Build history of the part. All positions in model axes, mm. A direction names the side the tool comes from. Give positions to 0.01 mm unless a question says otherwise; leave off trailing zeros. Loops run counter-clockwise (first coordinate to the right, second up) from the corner with the lowest first, then second, coordinate; pieces in that order, holes last. Notation, with made-up numbers: (-38.5, 55) - (-26.5, 55) arc R18 ccw to (-26.5, 60) - close; hole circle Ø1 at (-27, 7). An arc over 180 degrees is marked (long way). Return JSON: item names as keys, results as strings. Group by question number.
1) 3-axis set-ups, long thin cutter, end or side, ignore diameter. For faces 4 (the face through (-1, 2.641, 64)), 5 (the face through (39.531, 0, 40)), 6 (the face through (-1, -6.109, 40)), 7 (the face through (-1, 6.109, 40)), 8 (the face through (-39.531, 0, 40)): which of +Z, -Z, +X, -X, +Y, -Y reach the whole face in a straight line?
2) Slice it at D-D (x = 0). List the corners of the cut face in (y, z).
3) Drop flat-ended pins along their axis: pin 1 (3 mm diameter, centred on x = -2.5, z = 21.5, fed in from +Y); pin 2 (13.5 mm diameter, centred on y = -1, z = 37, fed in from +X); pin 3 (1.5 mm diameter, centred on y = -23.5, z = 7, fed in from -X); pin 4 (7 mm diameter, centred on x = -21.57, z = 27.49, fed in from -Y). Give the stop position or say it passes through.
4) Slice it at A-A (x = -17.5). List the corners of the cut face in (y, z).
5) Mould opens along Z. For faces 1 (the face through (-17.1, 0.1, 31.5)), 2 (the face through (-1, 0, 62)), 3 (the face through (-1, 1, 0)) say: released by +Z, released by -Z, zero draft, split by the parting line, or undercut.
6) Slice it at C-C (z = 24). List the corners of the cut face in (x, y), and give its area (3 significant figures).
7) Slice it at B-B (y = 0). List the corners of the cut face in (x, z).
8) Drill centre lines: probe 1 along X at (y, z) = (-1.5, 28); probe 2 along Y at (x, z) = (0.5, 17); probe 3 along X at (y, z) = (-1.5, 47.5). Where is each one in solid material? Low to high. Write a range as from..to.
```python
from build123d import *

# Parameters (mm, degrees)
F0_R     = 40
F1_DEPTH = 15
F2_W     = 79.06135
F2_H     = 12.21896
F3_DEPTH = 50
F4_W     = 79.06135
F4_H     = 5.281066
F5_DEPTH = 3
F6_R     = 6
F7_DEPTH = 25


with BuildPart() as f1:
    # F0 (on Top) → F1 (new body)
    with BuildSketch(Plane.XY):
        Circle(F0_R)
    extrude(amount=F1_DEPTH)

    # F2 (on face) → F3 (join)
    with BuildSketch(Plane.XY.offset(15)):
        Rectangle(F2_W, F2_H)
    extrude(amount=F3_DEPTH)

    # F4 (on face) → F5 (cut)
    with BuildSketch(Plane.XY.offset(65)):
        Rectangle(F4_W, F4_H)
    extrude(amount=-F5_DEPTH, mode=Mode.SUBTRACT)

    # F6 (on face) → F7 (cut)
    with BuildSketch(Plane(origin=(0, 6.10948, 0), x_dir=(-1, 0, 0), z_dir=(0, 1, 0))):
        with Locations((-21.04659, 27.803255)):
            Circle(F6_R)
        with Locations((21.568101, 27.492605)):
            Circle(F6_R)
    extrude(amount=-F7_DEPTH, mode=Mode.SUBTRACT)


solid = f1.part
```
Results:
{
 "1": {"face 4": "+Z, +X, -X", "face 5": "+Z, +X, +Y, -Y", "face 6": "+Z, +X, -X, -Y", "face 7": "+Z, +X, -X, +Y", "face 8": "+Z, -X, +Y, -Y"},
 "2": {"outline": "(-40, 0) - (40, 0) - (40, 15) - (6.11, 15) - (6.11, 65) - (2.64, 65) - (2.64, 62) - (-2.64, 62) - (-2.64, 65) - (-6.11, 65) - (-6.11, 15) - (-40, 15) - close"},
 "3": {"pin 1": "y = 6.11", "pin 2": "x = 39.53", "pin 3": "x = -32.9", "pin 4": "through"},
 "4": {"outline": "(-35.97, 0) - (35.97, 0) - (35.97, 15) - (6.11, 15) - (6.11, 23.08) - (-6.11, 23.08) - (-6.11, 15) - (-35.97, 15) - close; (-6.11, 31.9) - (6.11, 31.9) - (6.11, 65) - (2.64, 65) - (2.64, 62) - (-2.64, 62) - (-2.64, 65) - (-6.11, 65) - close"},
 "5": {"face 1": "undercut", "face 2": "released by +Z", "face 3": "released by -Z"},
 "6": {"outline": "(-39.53, -6.11) - (-26.45, -6.11) - (-26.45, 6.11) - (-39.53, 6.11) - close; (-16.69, -6.11) - (16.41, -6.11) - (16.41, 6.11) - (-16.69, 6.11) - close; (25.69, -6.11) - (39.53, -6.11) - (39.53, 6.11) - (25.69, 6.11) - close", "area": "733 mm2"},
 "7": {"outline": "(-40, 0) - (40, 0) - (40, 15) - (39.53, 15) - (39.53, 62) - (-39.53, 62) - (-39.53, 15) - (-40, 15) - close; hole circle Ø12 at (-21.57, 27.49); hole circle Ø12 at (21.05, 27.8)"},
 "8": {"probe 1": "-39.53..-27.55, -15.59..15.05, 27.04..39.53", "probe 2": "-6.11..6.11", "probe 3": "-39.53..39.53"}
}
